Here's how the part is built. I have some questions about the finished solid (model axes, mm). A direction names the side the tool comes from. Coordinates: 2 decimals unless noted, no trailing zeros. Order: outer loops, then holes, each group sorted by start corner. A loop starts at its lowest first (then second) coordinate and runs counter-clockwise, first axis right, second up. Notation, with made-up numbers: (45, -21) - (84, -21) arc R32 cw to (84, 12) - close; hole circle Ø5 at (-38, -10). An arc over 180 degrees is marked (long way). Answer in a Markdown table with one row per item. Add a question column.
Item 1: Thinking about a two-plate mould opening in X: for faces 4 (the cylindrical face through (-2.17, -9.76, 12.32)), 5 (the flat face through (2, 5, 25)), 6 (the cylindrical face through (1.08, -4.88, 4.93)), which applies, +X half, -X half, draft (parallel to the pull), parting line (faces both ways), or undercut?
Item 2: Will these pins go through, and if not, where does the flat tip stop? pin 1 Ø5 at (x, z) = (-6, 30) entering from +Y; pin 2 Ø2 at (y, z) = (5, 28.5) entering from -X; pin 3 Ø8 at (y, z) = (7, 34.5) entering from -X.
Item 3: If I drill on line 1 along Y through (x, z) = (0, 4.25); line 2 along Y through (x, z) = (0, 34.25); line 3 along Z through (x, y) = (5.75, 5.5), over which ranges is the centre line in solid material (lowest first)? Write a range as from..to.
Item 4: On a 3-axis mill with a long thin cutter (end or side, diameter ignored), from which of +Z, -Z, +X, -X, +Y, -Y can I reach the whole of each face in a straight line? I mean faces 1 (the cylindrical face through (5, 0, 33)), 2 (the flat face through (-5, -2, 0)), 3 (the flat face through (0, 0, 10)). Say none if no direction works.
Item 5: I want a section at D-D (z = 24). Please give me the cut outline in (x, y).
Item 6: I want a section at A-A (x = 0). Please give me the cut outline in (y, z).
Item 7: I want a section at B-B (z = 3.5). Please give me the cut outline in (x, y), plus the area to 3 significant figures.
```python
from build123d import *

# Parameters (mm, degrees)
SKETCH1_R           = 10
BOSS_EXTRUDE1_DEPTH = 41
SKETCH2_R           = 5
CUT_EXTRUDE1_DEPTH  = 10
SKETCH3_OUTSIDE_W   = 31.962
SKETCH3_OUTSIDE_H   = 31.962
SKETCH3_OUTSIDE_R   = 5
CUT_EXTRUDE2_DEPTH  = 16
SKETCH4_R           = 3.5
CUT_EXTRUDE3_DEPTH  = 12


with BuildPart() as part:
    # Sketch1 → Boss-Extrude1 (new body)
    with BuildSketch(Plane.XY):
        Circle(SKETCH1_R)
    extrude(amount=BOSS_EXTRUDE1_DEPTH)

    # Sketch2 → Cut-Extrude1 (cut)
    with BuildSketch(Plane(origin=(0, 0, 0), x_dir=(-1, 0, 0), z_dir=(0, 0, -1))):
        Circle(SKETCH2_R)
    extrude(amount=-CUT_EXTRUDE1_DEPTH, mode=Mode.SUBTRACT)

    # Sketch3 outside → Cut-Extrude2 (cut)
    with BuildSketch(Plane.XY.offset(41)):
        Rectangle(SKETCH3_OUTSIDE_W, SKETCH3_OUTSIDE_H)
        with Locations(Location((0, 0, 0), (0, 0, 180))):
            Circle(SKETCH3_OUTSIDE_R, mode=Mode.SUBTRACT)
    extrude(amount=-CUT_EXTRUDE2_DEPTH, mode=Mode.SUBTRACT)

    # Sketch4 → Cut-Extrude3 (cut)
    with BuildSketch(Plane.XY.offset(41)):
        Circle(SKETCH4_R)
    extrude(amount=-CUT_EXTRUDE3_DEPTH, mode=Mode.SUBTRACT)


solid = part.part
```
Values follow:
| question | item | result |
|---|---|---|
| 1 | face 4 | parting line |
| 1 | face 5 | draft |
| 1 | face 6 | undercut |
| 2 | pin 1 | stops at y = 3.57 |
| 2 | pin 2 | stops at x = -3 |
| 2 | pin 3 | stops at x = -4 |
| 3 | line 1 | y = -10..-5, 5..10 |
| 3 | line 2 | y = -5..-3.5, 3.5..5 |
| 3 | line 3 | z = 0..25 |
| 4 | face 1 | +Z |
| 4 | face 2 | -Z, +X, -X, +Y, -Y |
| 4 | face 3 | -Z |
| 5 | outline | circle Ø20 at (0, 0) |
| 6 | outline | (-10, 0) - (-5, 0) - (-5, 10) - (5, 10) - (5, 0) - (10, 0) - (10, 25) - (5, 25) - (5, 41) - (3.5, 41) - (3.5, 29) - (-3.5, 29) - (-3.5, 41) - (-5, 41) - (-5, 25) - (-10, 25) - close |
| 7 | outline | circle Ø20 at (0, 0); hole circle Ø10 at (0, 0) |
| 7 | area | 236 mm^2 |
